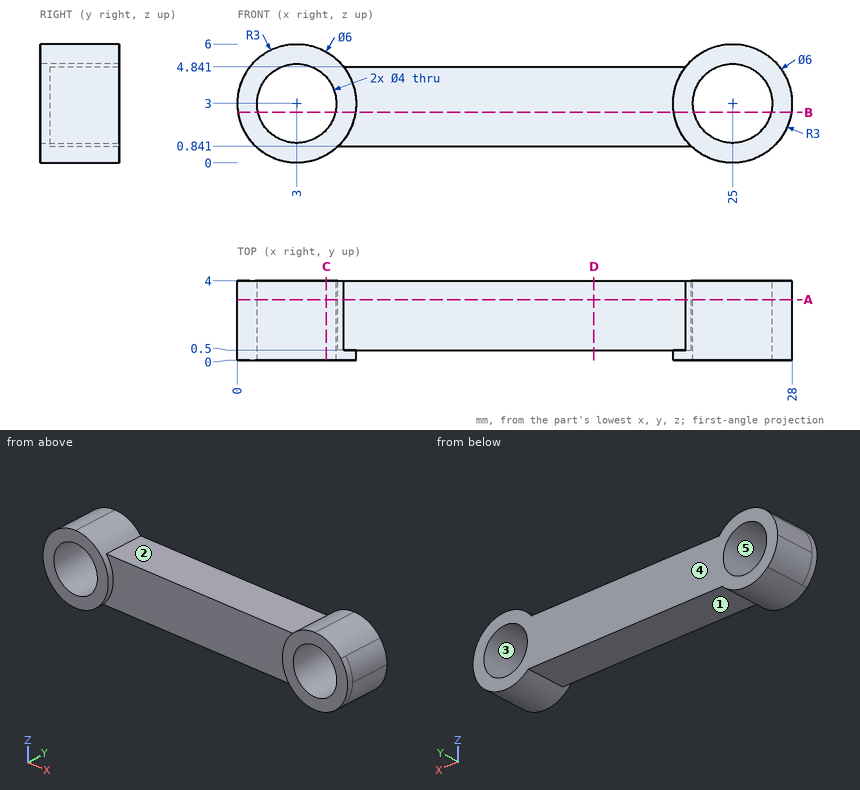
Source: three-view drawing plus pictorial views. Frame: mm from the lowest corner of the part. A direction names the side the tool comes from. Give positions to 0.01 mm unless a question says otherwise; leave off trailing zeros. Loops run counter-clockwise (first coordinate to the right, second up) from the corner with the lowest first, then second, coordinate; pieces in that order, holes last.
1) Section query A-A on y = 3.05. Return the cut outline in (x, z).
A:
outline: (5.08, 0.84) - (22.92, 0.84) arc R3 ccw (long way) to (22.63, 4.84) - (5.37, 4.84) arc R3 ccw (long way) to start; hole circle Ø4 at (3, 3); hole circle Ø4 at (25, 3)
2) Line query: L1, parallel to X at y = 1.45, z = 3.1; L2, parallel to Y at x = 18, z = 2.55; L3, parallel to X at y = 3.1, z = 3.85. Output: solid intervals per line, ascending.
A:
L1: x = 0 to 1, 5 to 23, 27 to 28
L2: y = 0.5 to 4
L3: x = 0.12 to 1.19, 4.81 to 23.19, 26.81 to 27.88
3) Section query D-D on x = 18. Return the cut outline in (y, z), and give its area (3 significant figures).
A:
outline: (0.5, 0.84) - (4, 0.84) - (4, 4.84) - (0.5, 4.84) - close
area: 14.0 mm2
4) Reachability of the marked faces 1, 2 and 3 from +Z, -Z, +X, -X, +Y, -Y: full face, straight path, thin tool, end or side. Return the list, or none.
A:
face 1: -Z, +Y, -Y
face 2: +Z, +Y, -Y
face 3: +Y, -Y
5) Contact query for flat-ended pins moving along their axis: pin 1 (1.5 mm diameter, centred on x = 15.5, y = 1, fed in from -Z); pin 2 (1.5 mm diameter, centred on x = 24, y = 2, fed in from +Z); pin 3 (1.8 mm diameter, centred on x = 13.5, y = 3, fed in from +Z). Output: stop coordinate, or through.
A:
pin 1: stops at z = 0.84
pin 2: stops at z = 5.99
pin 3: stops at z = 4.84
6) Section query C-C on x = 4.5. Return the cut outline in (y, z).
A:
outline: (0, 0.4) - (4, 0.4) - (4, 1.68) - (0, 1.68) - close; (0, 4.32) - (4, 4.32) - (4, 5.6) - (0, 5.6) - close
7) Mould query, pull axis X, two halves, no side actions, for the marked faces 4 and 5. Classes: released by +X, released by -X, zero draft, split by the parting line, or undercut.
A:
face 4: zero draft
face 5: undercut
8) Section query B-B on z = 2.55. Return the cut outline in (x, y).
A:
outline: (0.03, 0) - (1.05, 0) - (1.05, 4) - (0.03, 4) - close; (4.95, 0) - (5.97, 0) - (5.97, 0.5) - (22.03, 0.5) - (22.03, 0) - (23.05, 0) - (23.05, 4) - (4.95, 4) - close; (26.95, 0) - (27.97, 0) - (27.97, 4) - (26.95, 4) - close
